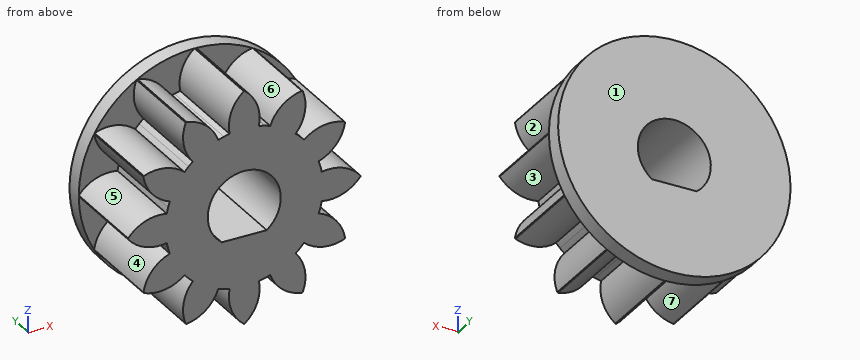
from build123d import *

# Parameters (mm, degrees)
BOSS_EXTRUDE2_DEPTH = 8
CIRPATTERN4_COUNT   = 12
CUT_EXTRUDE1_DEPTH  = 17.867127793
SKETCH8_R           = 10.5
BOSS_EXTRUDE3_DEPTH = 1.5


with BuildPart() as part:
    # Sketch6 → Boss-Extrude2 (new body)
    with BuildSketch(Plane(origin=(0, 0, 0), x_dir=(-1, 0, 0), z_dir=(0, 1, 0))):
        with BuildLine():
            Line((-1.844085696, 6.882221512), (-0.258819045, 0.965925826))
            ThreePointArc((-0.258819045, 0.965925826), (0, 1), (0.258819045, 0.965925826))
            Line((0.258819045, 0.965925826), (1.844085696, 6.882221512))
            ThreePointArc((1.844085696, 6.882221512), (1.585602155, 6.946329305), (1.324903403, 7.000732531))
            ThreePointArc((1.324903403, 7.000732531), (1.172594993, 8.928869546), (0.0444307, 10.499905995))
            ThreePointArc((0.0444307, 10.499905995), (0, 10.5), (-0.0444307, 10.499905995))
            ThreePointArc((-0.0444307, 10.499905995), (-1.172594993, 8.928869546), (-1.324903403, 7.000732531))
            ThreePointArc((-1.324903403, 7.000732531), (-1.585602155, 6.946329305), (-1.844085696, 6.882221512))
        make_face()
    boss_extrude2 = extrude(amount=BOSS_EXTRUDE2_DEPTH)

    # CirPattern4: Boss-Extrude2 ×12 about axis
    cirpattern4_axis = Axis((0, 0, 0), (0, 1, 0))
    for i in range(1, CIRPATTERN4_COUNT):
        add(boss_extrude2.rotate(cirpattern4_axis, i * 360 / CIRPATTERN4_COUNT))

    # Sketch7 → Cut-Extrude1 (cut, through all)
    with BuildSketch(Plane(origin=(0, 8, 0), x_dir=(1, 0, 0), z_dir=(0, 1, 0))):
        with BuildLine():
            Line((2.032240143, 2.6), (-2.032240143, 2.6))
            ThreePointArc((-2.032240143, 2.6), (0, -3.3), (2.032240143, 2.6))
        make_face()
    extrude(amount=-CUT_EXTRUDE1_DEPTH, mode=Mode.SUBTRACT)

    # Sketch8 → Boss-Extrude3 (add)
    with BuildSketch(Plane(origin=(0, 8, 0), x_dir=(1, 0, 0), z_dir=(0, 1, 0))):
        with Locations(Location((0, 0, 0), (0, 0, 89.757552457))):
            Circle(SKETCH8_R)
        with BuildLine():
            Line((2.032240143, 2.6), (-2.032240143, 2.6))
            ThreePointArc((-2.032240143, 2.6), (0, -3.3), (2.032240143, 2.6))
        make_face(mode=Mode.SUBTRACT)
    extrude(amount=BOSS_EXTRUDE3_DEPTH)


solid = part.part
Here's how the part is built. I have some questions about the finished solid (model axes, mm). Face numbers are marked on the shaded views. A direction names the side the tool comes from. Round coordinates to 2 decimals unless told otherwise and drop trailing zeros. Loops run counter-clockwise (first coordinate to the right, second up) from the corner with the lowest first, then second, coordinate; pieces in that order, holes last. Notation, with made-up numbers: M 15,74 L 40,74 A11 cw 40,85 Z; hole C 17.25,15 d11. An arc over 180 degrees is marked long. Write each question's results on one line, items separated by ' | '. Start each with the question number.
(1) Will these pins go through, and if not, where does the flat tip stop? P1, Ø1.9, axis at x = -3, z = 9, coming from the -Y side; P2, Ø4, axis at x = 2.5, y = 2, coming from the -Z side; P3, Ø2, axis at x = 6.5, z = -7, coming from the -Y side; P4, Ø1.5, axis at y = 8.5, z = -4.5, coming from the -X side.
(2) I want a section at C-C (x = -7.5). Please give me the cut outline in (y, z), then the cut area to 3 significant figures.
(3) I want a section at A-A (x = 3.75). Please give me the cut outline in (y, z) (3 decimals), then the cut area to 3 significant figures.
(4) I want a section at B-B (z = 8.5). Please give me the cut outline in (x, y), then the cut area to 3 significant figures.
(5) If I drill on probe 1 along X at (y, z) = (4, 0); probe 2 along Z at (x, y) = (8, 4); probe 3 along Z at (x, y) = (8.25, 1.5), over which ranges is the centre line in solid material (lowest first)? Write a range as from..to.
(6) I want a section at D-D (z = -6). Please give me the cut outline in (x, y).
(7) On a 3-axis mill with a long thin cutter (end or side, diameter ignored), from which of +Z, -Z, +X, -X, +Y, -Y can I reach the whole of each face in a straight line? I mean the marked faces 1, 2, 3 and 4. Say none if no direction works.
(8) Thinking about a two-plate mould opening in Z: for the marked faces 5, 6 and 7, which applies, pulls with the +Z half, pulls with the -Z half, needs draft (parallel to the pull), parting line crosses it, or undercut?
Solved:
1) P1: stops at y = 0 | P2: stops at z = -10.06 | P3: stops at y = 8 | P4: stops at x = -9.81
2) outline: M 0,-5.52 L 8,-5.52 L 8,-7.35 L 9.5,-7.35 L 9.5,7.35 L 8,7.35 L 8,5.52 L 0,5.52 L 0,2.73 L 8,2.73 L 8,1.39 L 0,1.39 L 0,-1.39 L 8,-1.39 L 8,-2.73 L 0,-2.73 Z | area: 89.0 mm²
3) outline: M 0,-8.545 L 8,-8.545 L 8,-9.808 L 9.5,-9.808 L 9.5,9.808 L 8,9.808 L 8,8.545 L 0,8.545 Z | area: 166 mm²
4) outline: M -6.16,8 L -5.46,8 L -5.46,0 L -3.68,0 L -3.68,8 L -1.3,8 L -1.3,0 L 1.3,0 L 1.3,8 L 3.68,8 L 3.68,0 L 5.46,0 L 5.46,8 L 6.16,8 L 6.16,9.5 L -6.16,9.5 Z | area: 67.7 mm²
5) probe 1: x = -10.5..-3.3, 3.3..10.5 | probe 2: z = -5.53..-3.11, -1.38..1.38, 3.11..5.53 | probe 3: z = -5.5..-3.37, -1.35..1.35, 3.37..5.5
6) outline: M -8.62,8 L -5.07,8 L -5.07,0 L 5.07,0 L 5.07,8 L 8.62,8 L 8.62,9.5 L -8.62,9.5 Z
7) face 1: +Z, -Z, +X, -X, +Y | face 2: +X, -Y | face 3: -Y | face 4: -X, -Y
8) face 5: undercut | face 6: pulls with the +Z half | face 7: pulls with the -Z half
